The listing builds one solid part. Answer for the finished solid, in the listing's coordinates (mm). A direction names the side the tool comes from. Round coordinates to 2 decimals unless told otherwise and drop trailing zeros. Loops run counter-clockwise (first coordinate to the right, second up) from the corner with the lowest first, then second, coordinate; pieces in that order, holes last. Notation, with made-up numbers: M 41,32 L 63,32 A31 ccw 63,68 Z; hole C 31,0 d3. An arc over 180 degrees is marked long. Answer as a JSON object with one key per item and string values.
```python
from build123d import *

# Parameters (mm, degrees)
F1_DEPTH = 26.416
F2_R     = 1.8415
F3_DEPTH = 2.54
F7_DEPTH = 7.62


with BuildPart() as f1:
    # F0 (on Front) → F1 (new body)
    with BuildSketch(Plane.XZ):
        with BuildLine():
            Line((-4.9881667079, -6.5078052628), (18.9825711812, -6.5078052628))
            Line((18.9825711812, -6.5078052628), (18.9825711812, -3.9678052628))
            Line((18.9825711812, -3.9678052628), (-5.5439422008, -2.3553312877))
            ThreePointArc((-5.5439422008, -2.3553312877), (-5.9622258253, -2.2601628666), (-6.3636870308, -2.1090102306))
            Line((-6.3636870308, -2.1090102306), (-11.9552752015, 0.4437738695))
            ThreePointArc((-11.9552752015, 0.4437738695), (-14.6813052169, -0.5733543796), (-13.6641769678, -3.299384395))
            Line((-13.6641769678, -3.299384395), (-8.0725887971, -5.8521684951))
            ThreePointArc((-8.0725887971, -5.8521684951), (-6.5663902888, -6.3494066979), (-4.9881667079, -6.5078052628))
        make_face()
    extrude(amount=F1_DEPTH)

    # F2 (on face) → F3 (join)
    with BuildSketch(Plane.XZ.offset(26.416)):
        with Locations((-12.8097260847, -1.4278052628)):
            Circle(F2_R)
    extrude(amount=F3_DEPTH)

    # F5: F1 across plane


with BuildPart() as f1_1:
    add(f1.part)
    add(f1.part.mirror(Plane(origin=(1.3145173971, -13.208, -4.2776395972), x_dir=(1, 0, 0), z_dir=(0, 1, 0))))


with BuildPart() as f7:
    # F6 (on face) → F7 (new body, symmetric)
    with BuildSketch(Plane(origin=(0, 0, -6.5078052628), x_dir=(1, 0, 0), z_dir=(0, 0, -1))):
        Polygon((-4.9881667079, 23.4607403946), (-16.556808725, 24.4735703084), (-16.556808725, 1.9424296916), (-4.9881667079, 2.9552596054), align=None)
        with BuildLine():
            Line((4.2894943617, 22.648484933), (-4.9881667079, 23.4607403946))
            Line((-4.9881667079, 23.4607403946), (-4.9881667079, 2.9552596054))
            Line((-4.9881667079, 2.9552596054), (4.2894943617, 3.767515067))
            ThreePointArc((4.2894943617, 3.767515067), (12.9395799393, 13.208), (4.2894943617, 22.648484933))
        make_face()
    extrude(amount=F7_DEPTH, both=True)


with BuildPart() as f1_2:
    add(f1_1.part)

    # F8: cut F7
    add(f7.part, mode=Mode.SUBTRACT)


solid = f1_2.part
```
Item 1: The part is cut by section B-B (y = -1). Give the vertices of the cut face in (x, z), then the cut area to 3 significant figures.
Values follow:
{"outline": "M -13.66,-3.3 L -8.07,-5.85 A7.26 ccw -4.99,-6.51 L 18.98,-6.51 L 18.98,-3.97 L -5.54,-2.36 A3.15 cw -6.36,-2.11 L -11.96,0.44 A2.06 ccw Z", "area": "121 mm^2"}
Item 2: Which of the six approach directions +Z, -Z, +X, -X, +Y, -Y give full straight-line access (tool end or side, diameter ignored) to faces 1 (the face through (-11.053, 1.252, -0.875)), 2 (the face through (-11.053, -27.668, -0.875)), 3 (the face through (15, -13, -6.508))?
Values follow:
{"face 1": "+Y", "face 2": "-Y", "face 3": "-Z, +X, -X, +Y, -Y"}
Item 3: The part is cut by section C-C (x = -2.5). Give the vertices of the cut face in (y, z), then the cut area to 3 significant figures.
Values follow:
{"outline": "M -26.42,-6.51 L -23.24,-6.51 L -23.24,-2.56 L -26.42,-2.56 Z; M -3.17,-6.51 L 0,-6.51 L 0,-2.56 L -3.17,-2.56 Z", "area": "25.1 mm^2"}
Item 4: Straight lines are drawn through the part: line 1 (Y direction, x = 9.5, z = -3.5); line 2 (Z direction, x = 3.5, y = -24); line 3 (Y direction, x = 6, z = -3.5). For each, find the intervals that lie inside material, in ascending order.
Values follow:
{"line 1": "-26.42 to -20.51, -5.9 to 0", "line 2": "-6.51 to -2.95", "line 3": "-26.42 to -22.34, -4.08 to 0"}
Item 5: The part is cut by section D-D (x = 16.5). Give the vertices of the cut face in (y, z), then the cut area to 3 significant figures.
Values follow:
{"outline": "M -26.42,-6.51 L 0,-6.51 L 0,-3.8 L -26.42,-3.8 Z", "area": "71.4 mm^2"}
Item 6: The part is cut by section A-A (x = 3.5). Give the vertices of the cut face in (y, z).
Values follow:
{"outline": "M -26.42,-6.51 L -22.72,-6.51 L -22.72,-2.95 L -26.42,-2.95 Z; M -3.7,-6.51 L 0,-6.51 L 0,-2.95 L -3.7,-2.95 Z"}
Item 7: Flat-ended cylindrical pins translate along their axes: P1, Ø5, axis at x = -2, y = -24, coming from the +Z side; P2, Ø6, axis at x = 2, y = -22.5, coming from the +Z side; P3, Ø1, axis at y = -12.5, z = -5.5, coming from the -X side; P4, Ø2, axis at x = 14.5, z = -1, coming from the -Y side. Find the tip coordinate at first contact, or state that the pin passes through.
Values follow:
{"P1": "z = -2.42", "P2": "z = -2.66", "P3": "x = 12.86", "P4": "through"}
